Autodesk Inventor part; units mm, degrees
ref_plane "YZ Plane" through (0, 0, 0) normal (1, 0, 0) x (0, 1, 0)
ref_plane "XZ Plane" through (0, 0, 0) normal (0, 1, 0) x (-1, 0, 0)
ref_plane "XY Plane" through (0, 0, 0) normal (0, 0, 1) x (1, 0, 0)
sketch "Esboço1" plane through (0, 0, 0) normal (0, 0, 1) x (1, 0, 0)
  circle A0 centre (0, 0) radius 8
  dimension "d0" = 16
extrude "Extrusão1" add sketch "Esboço1" along normal blind 30
sketch "Esboço2" plane through (0, 0, 30) normal (0, 0, 1) x (1, 0, 0)
  circle A0 centre (0, 0) radius 6
  dimension "d3" = 12
extrude "Extrusão2" add sketch "Esboço2" along normal blind 39
sketch "Esboço3" plane through (0, 0, 69) normal (0, 0, 1) x (1, 0, 0)
  circle A0 centre (0, 0) radius 5
  dimension "d6" = 10
extrude "Extrusão3" add sketch "Esboço3" along normal blind 15
sketch "Esboço4" plane through (0, 0, 0) normal (0, 0, -1) x (-1, 0, 0)
  circle A0 centre (0, 0) radius 5
  dimension "d9" = 10
extrude "Extrusão4" add sketch "Esboço4" along normal blind 9.15
sketch "Esboço5" plane through (0, 0, -9.15) normal (0, 0, -1) x (-1, 0, 0)
  circle A0 centre (0, 0) radius 4.5
  dimension "d12" = 9
extrude "Extrusão5" add sketch "Esboço5" along normal blind 1.15
sketch "Esboço6" plane through (0, 0, -10.3) normal (0, 0, -1) x (-1, 0, 0)
  circle A0 centre (0, 0) radius 5
  dimension "d15" = 10
extrude "Extrusão6" add sketch "Esboço6" along normal blind 1.85
thread "Rosca1"
chamfer "Chanfro1" distance 1 angle 45 5 edges at (-5, 0, 84) (-6, 0, 69) (-8, 0, 30) (-8, 0, 0) (5, 0, -12.15)
properties part number "SFU16XX"
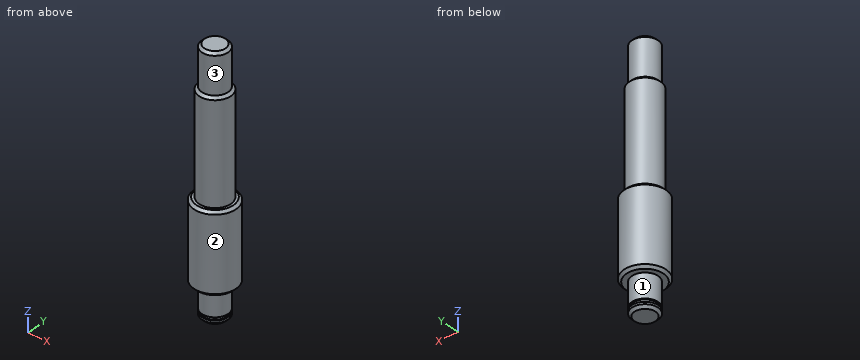
Build history of the part. All positions in model axes, mm. Face numbers are marked on the shaded views. A direction names the side the tool comes from. Round coordinates to 2 decimals unless told otherwise and drop trailing zeros. Write each loop counter-clockwise with the first axis right and the second up, starting at its lowest first coordinate (ties: lowest second). Pieces come first, ordered by that corner, then holes. Notation, with made-up numbers: M -13,-23 L 14,-23 A30 ccw 14,8 Z; hole C -6,-7 d3. An arc over 180 degrees is marked long. Answer as a JSON object with one key per item and string values. Group by question number.
(1) Cut at D-D (z = 77). Give the cut face in (x, y), and give its area (3 significant figures).
(2) Cut at C-C (z = 48.5). Give the cut face in (x, y).
(3) Flat gauge pins, fed straight in: pin 1 (3 mm diameter, centred on y = -4.5, z = 40.5, fed in from +X); pin 2 (5 mm diameter, centred on x = 5.5, z = 34, fed in from +Y); pin 3 (4 mm diameter, centred on y = 3, z = 28.5, fed in from -X). Where does each tip first touch, or does it go through?
(4) Drill centre lines: L1, parallel to Y at x = -6.25, z = 26.5; L2, parallel to Z at x = 4.75, y = 4.25; L3, parallel to Z at x = -1, y = -7. Where is each one in solid material? Low to high.
(5) Which spindle directions (+Z, -Z, +X, -X, +Y, -Y) get a long thin tool onto all of the face, cutting with end or side? Do the marked faces 1, 2 and 3. Say none if no direction does.
Responses:
{
 "1": {"outline": "C 0,0 d10", "area": "78.5 mm2"},
 "2": {"outline": "C 0,0 d12"},
 "3": {"pin 1": "stops at x = 5.2", "pin 2": "stops at y = 5.2", "pin 3": "stops at x = -7.94"},
 "4": {"L1": "y = -4.99 to 4.99", "L2": "z = 0 to 30", "L3": "z = 0.07 to 29.93"},
 "5": {"face 1": "-Z", "face 2": "+Z, -Z", "face 3": "+Z"}
}
